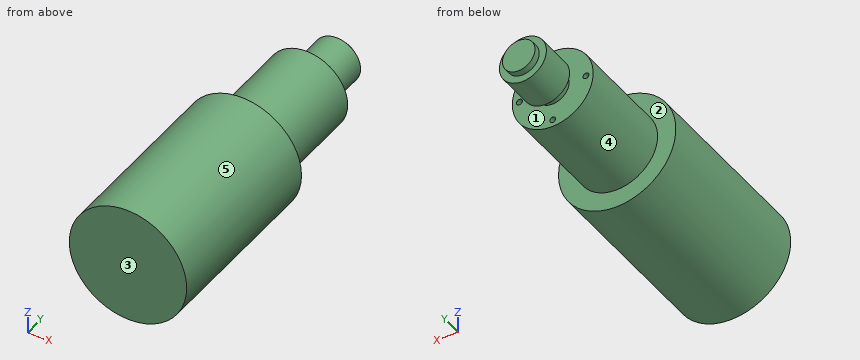
from build123d import *

# Parameters (mm, degrees)
FORO_PER_VITE_M4_1_D           = 4.5
FORO_PER_VITE_M4_1_DEPTH       = 17
FORO_PER_VITE_M4_1_CSINK_D     = 4.55
FORO_PER_VITE_M4_1_CSINK_ANGLE = 90
FORO_PER_VITE_M4_1_TIP         = 1.351936393


with BuildPart() as part:
    # Schizzo2 → Rivoluzione1 (revolve)
    with BuildSketch(Plane.XY):
        Polygon((0, 257.3), (12.5, 257.3), (12.5, 252.3), (18, 252.3), (18, 224.3), (12.5, 224.3), (12.5, 216.3), (31, 216.3), (31, 138.55), (45, 138.55), (45, 0), (0, 0), align=None)
    revolve(axis=Axis((0, -1182.394203663, 0), (0, 1, 0)))

    # Foro per Vite M4-1
    with Locations(Plane(origin=(0, 216.3, 0), x_dir=(1, 0, 0), z_dir=(0, 1, 0))):
        with Locations((0, 25.5), (25.5, 0), (0, -25.5), (-25.5, 0)):
            CounterSinkHole(FORO_PER_VITE_M4_1_D / 2, FORO_PER_VITE_M4_1_CSINK_D / 2, depth=FORO_PER_VITE_M4_1_DEPTH, counter_sink_angle=FORO_PER_VITE_M4_1_CSINK_ANGLE)
            with Locations((0, 0, -(FORO_PER_VITE_M4_1_DEPTH + FORO_PER_VITE_M4_1_TIP / 2))):  # 118° drill point
                Cone(0, FORO_PER_VITE_M4_1_D / 2, FORO_PER_VITE_M4_1_TIP, mode=Mode.SUBTRACT)


solid = part.part
Geometry check sheet. Reference: the model listing, model coordinates, mm. Face numbers are marked on the shaded views. A direction names the side the tool comes from. Give positions to 0.01 mm unless a question says otherwise; leave off trailing zeros. Order: outer loops, then holes, each group sorted by start corner. A loop starts at its lowest first (then second) coordinate and runs counter-clockwise, first axis right, second up. Notation, with made-up numbers: M -3,50 L 43,50 A22 ccw 43,87 Z; hole C 75,-36.75 d8. An arc over 180 degrees is marked long. Use a Markdown table: item, result.
Item 1: Section check A-A (y = 174). Record the cut outline in (x, z).
Answers follow:
| item | result |
|---|---|
| outline | C 0,0 d62 |
Item 2: Section check C-C (z = 7). Record the cut outline in (x, y).
Answers follow:
| item | result |
|---|---|
| outline | M -44.45,0 L 44.45,0 L 44.45,138.55 L 30.2,138.55 L 30.2,216.3 L 10.36,216.3 L 10.36,224.3 L 16.58,224.3 L 16.58,252.3 L 10.36,252.3 L 10.36,257.3 L -10.36,257.3 L -10.36,252.3 L -16.58,252.3 L -16.58,224.3 L -10.36,224.3 L -10.36,216.3 L -30.2,216.3 L -30.2,138.55 L -44.45,138.55 Z |
Item 3: Section check D-D (y = 130). Record the cut outline in (x, z), and give its area (3 significant figures).
Answers follow:
| item | result |
|---|---|
| outline | C 0,0 d90 |
| area | 6,360 mm2 |
Item 4: Section check B-B (z = -9.5). Record the cut outline in (x, y), and give its area (3 significant figures).
Answers follow:
| item | result |
|---|---|
| outline | M -43.99,0 L 43.99,0 L 43.99,138.55 L 29.51,138.55 L 29.51,216.3 L 8.12,216.3 L 8.12,224.3 L 15.29,224.3 L 15.29,252.3 L 8.12,252.3 L 8.12,257.3 L -8.12,257.3 L -8.12,252.3 L -15.29,252.3 L -15.29,224.3 L -8.12,224.3 L -8.12,216.3 L -29.51,216.3 L -29.51,138.55 L -43.99,138.55 Z |
| area | 17,800 mm2 |
Item 5: Draft check along Y on the marked faces 1, 2 and 3. Enter one of: +Y half, -Y half, draft (parallel to the pull), parting line (faces both ways), or undercut.
Answers follow:
| item | result |
|---|---|
| face 1 | undercut |
| face 2 | +Y half |
| face 3 | -Y half |
Item 6: Tool access check on the marked faces 4 and 5. Record the directions out of +Z, -Z, +X, -X, +Y, -Y that give a thin tool (end or side, any length) a straight path to the whole face; none if there is none.
Answers follow:
| item | result |
|---|---|
| face 4 | +Y |
| face 5 | +Y, -Y |
Item 7: Material ranges on line 1 along Z through (x, y) = (0, 206.5); line 2 along Y through (x, z) = (-3, -16.5); line 3 along Y through (x, z) = (19.5, 12.5), recorded low to high.
Answers follow:
| item | result |
|---|---|
| line 1 | z = -31 to -27.75, -23.25 to 23.25, 27.75 to 31 |
| line 2 | y = 0 to 216.3, 224.3 to 252.3 |
| line 3 | y = 0 to 216.3 |
Item 8: Depth check by flat-ended pin: P1, Ø2, axis at y = 72.5, z = 4.5, coming from the +X side; P2, Ø10, axis at x = -11.5, y = 146.5, coming from the -Z side; P3, Ø12, axis at x = 35.5, z = -22, coming from the +Y side. Enter the tip coordinate at first touch or a pass-through.
Answers follow:
| item | result |
|---|---|
| P1 | stops at x = 44.86 |
| P2 | stops at z = -30.31 |
| P3 | stops at y = 138.55 |
